For this review, use the dimensioned drawing (mm, ordinates from the lowest corner) and the shaded views. Coordinates: 2 decimals unless noted, no trailing zeros. Loops run counter-clockwise (first coordinate to the right, second up) from the corner with the lowest first, then second, coordinate; pieces in that order, holes last. Notation, with made-up numbers: (17, -7) - (63, -7) arc R18 cw to (63, 6) - close; hole circle Ø7 at (88.25, 53). An arc over 180 degrees is marked (long way). Use one line per item in the form item = value. Start each with the question number.
(1) Add section B-B (y = 25). State the section outline as (x, z) points.
(2) Clearance check with flat-ended pins moving along their axes: pin 1 Ø1.5 at (x, z) = (158.5, 3) entering from -Y; pin 2 Ø2.5 at (x, z) = (157.5, 3) entering from +Y; pin 3 Ø1.5 at (y, z) = (43, 3.5) entering from +X. State where each tip first meets the part, or that it passes through.
(3) Add section A-A (z = 4). State the section outline as (x, y) points, plus the area to 3 significant figures.
(4) For L1, parallel to X at y = 29.5, z = 0.85; L2, parallel to X at y = 4, z = 3.2, list the stretches that pass through material, from the lowest coordinate up.
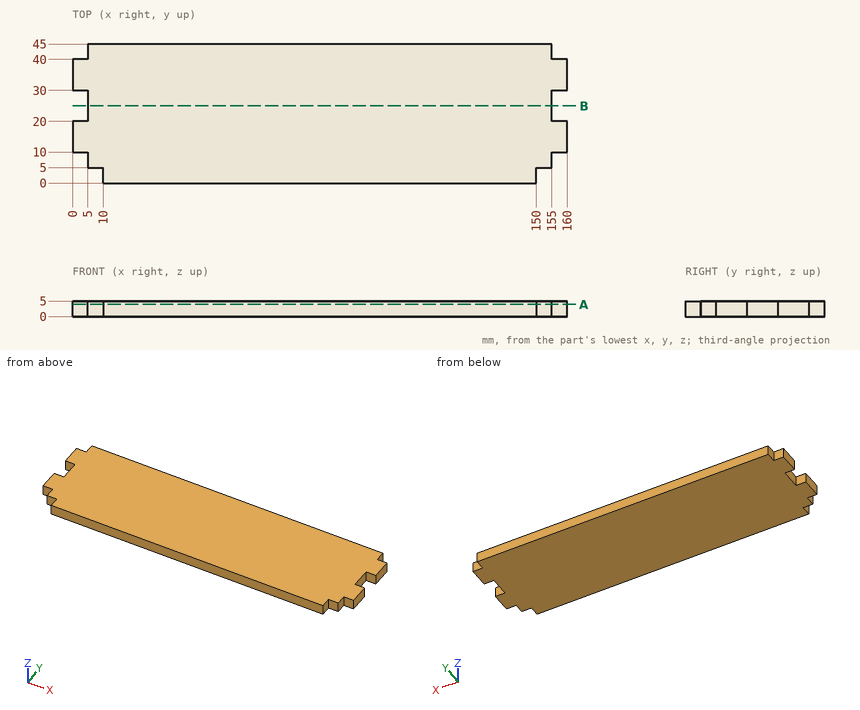
Computed values:
q1.outline = (5, 0) - (155, 0) - (155, 5) - (5, 5) - close
q2.pin_1 = 10
q2.pin_2 = 40
q2.pin_3 = 155
q3.outline = (0, 10) - (5, 10) - (5, 5) - (10, 5) - (10, 0) - (150, 0) - (150, 5) - (155, 5) - (155, 10) - (160, 10) - (160, 20) - (155, 20) - (155, 30) - (160, 30) - (160, 40) - (155, 40) - (155, 45) - (5, 45) - (5, 40) - (0, 40) - (0, 30) - (5, 30) - (5, 20) - (0, 20) - close
q3.area = 6,900 mm^2
q4.L1 = 5 to 155
q4.L2 = 10 to 150
